Check sheet for the modelled part. Datum: model origin and axes. Units: mm. A direction names the side the tool comes from. Give positions to 0.01 mm unless a question says otherwise; leave off trailing zeros. Loops run counter-clockwise (first coordinate to the right, second up) from the corner with the lowest first, then second, coordinate; pieces in that order, holes last. Notation, with made-up numbers: (-30.5, 11.25) -> (-24.5, 11.25) arc R6 cw to (-24.5, 15.25) -> close; hole circle Ø8 at (7.25, 9). An arc over 180 degrees is marked (long way). Answer as CSV lines item,"result". Start each with the question number.
(1) Gauge pin test, flat ends, axial feed: pin 1 Ø5 at (x, z) = (29.5, 310.5) entering from +Y; pin 2 Ø11.5 at (x, z) = (38.1, 12.7) entering from +Y. Record the tip position at first contact, or that the pin passes through.
(2) Section check C-C on z = 340.31. Enter the section's corners in (x, y) (3 decimals), plus the area to 3 significant figures.
(3) Access from +Z, -Z, +X, -X, +Y, -Y to the whole of each face (thin tool, end or side, straight path). Record for faces 4 (the face through (39.645, -3.944, 5.744)), 5 (the face through (24.684, -17.808, 345.763)).
(4) Section check A-A on x = 25.4. Enter the section's corners in (y, z) (3 decimals).
(5) Material ranges on line 1 (Z direction, x = 25.4, y = -20.25); line 2 (X direction, y = -3.75, z = 12.7) (3 decimals); line 3 (Z direction, x = 38.1, y = -4.25) (3 decimals), recorded low to high. Write a range as from..to.
(6) Section check B-B on y = -14. Enter the section's corners in (x, z), plus the area to 3 significant figures.
(7) Section check D-D on x = 6. Enter the section's corners in (y, z), plus the area to 3 significant figures.
(8) Release check for a two-part mould opening along Z. For faces 1 (the face through (26, -13, 400)), 2 (the face through (24.684, -17.808, 312.743)), 3 (the face through (0, -13, 203)) record: pulls with the +Z half, pulls with the -Z half, needs draft (parallel to the pull), parting line crosses it, or undercut.
from build123d import *

# Parameters (mm, degrees)
F1_DEPTH       = 25.4
F3_D           = 14.5
F5_D           = 8.8
F5_CBORE_D     = 14.25
F5_CBORE_DEPTH = 8
F7_D           = 11
F7_CBORE_D     = 17.25
F7_CBORE_DEPTH = 10


with BuildPart() as f1:
    # F0 (on Front) → F1 (new body)
    with BuildSketch(Plane.XZ):
        Polygon((0, 400), (0, 0), (76.2, 0), (76.2, 355.6), (50.8, 400), align=None)
    extrude(amount=F1_DEPTH)

    # F3 (through all)
    with Locations(Plane(origin=(0, 0, 0), x_dir=(0, -1, 0), z_dir=(-1, 0, 0))):
        with Locations((12.7, 20), (12.7, 380)):
            Hole(F3_D / 2)

    # F5 (through all)
    with Locations(Plane(origin=(0, 0, 0), x_dir=(-1, 0, 0), z_dir=(0, 1, 0))):
        with Locations((-63.5, 12.7), (-38.1, 12.7)):
            CounterBoreHole(F5_D / 2, F5_CBORE_D / 2, F5_CBORE_DEPTH)

    # F7 (through all)
    with Locations(Plane(origin=(0, 0, 0), x_dir=(-1, 0, 0), z_dir=(0, 1, 0))):
        with Locations((-25.4, 340.31), (-25.4, 307.29)):
            CounterBoreHole(F7_D / 2, F7_CBORE_D / 2, F7_CBORE_DEPTH)


solid = f1.part
Working result:
1,pin 1,"stops at y = -10"
1,pin 2,"stops at y = -8"
2,outline,"(0, -25.4) -> (19.9, -25.4) -> (19.9, -10) -> (16.775, -10) -> (16.775, 0) -> (0, 0) -> close; (30.9, -25.4) -> (76.2, -25.4) -> (76.2, 0) -> (34.025, 0) -> (34.025, -10) -> (30.9, -10) -> close"
2,area,"1,590 mm^2"
3,face 4,"+Y"
3,face 5,"+Y, -Y"
4,outline,"(-25.4, 0) -> (0, 0) -> (0, 298.665) -> (-10, 298.665) -> (-10, 301.79) -> (-25.4, 301.79) -> close; (-25.4, 312.79) -> (-10, 312.79) -> (-10, 315.915) -> (0, 315.915) -> (0, 331.685) -> (-10, 331.685) -> (-10, 334.81) -> (-25.4, 334.81) -> close; (-25.4, 345.81) -> (-10, 345.81) -> (-10, 348.935) -> (0, 348.935) -> (0, 400) -> (-25.4, 400) -> close; hole circle Ø14.5 at (-12.7, 20); hole circle Ø14.5 at (-12.7, 380)"
5,line 1,"z = 0..301.79, 312.79..334.81, 345.81..400"
5,line 2,"x = 0..30.975, 45.225..56.375, 70.625..76.2"
5,line 3,"z = 0..5.575, 19.825..400"
6,outline,"(0, 0) -> (76.2, 0) -> (76.2, 12.87) -> (67.9, 12.87) arc R4.4 cw (long way) to (59.1, 12.87) -> (42.5, 12.87) arc R4.4 cw (long way) to (33.7, 12.87) -> (0, 12.87) -> close; (0, 27.13) -> (76.2, 27.13) -> (76.2, 355.6) -> (66.32, 372.87) -> (0, 372.87) -> close; (0, 387.13) -> (58.16, 387.13) -> (50.8, 400) -> (0, 400) -> close; hole circle Ø11 at (25.4, 307.29); hole circle Ø11 at (25.4, 340.31)"
6,area,"27,700 mm^2"
7,outline,"(-25.4, 0) -> (0, 0) -> (0, 400) -> (-25.4, 400) -> close; hole circle Ø14.5 at (-12.7, 20); hole circle Ø14.5 at (-12.7, 380)"
7,area,"9,830 mm^2"
8,face 1,"pulls with the +Z half"
8,face 2,"undercut"
8,face 3,"needs draft"
